Source: three-view drawing plus pictorial views. Frame: mm from the lowest corner of the part. A direction names the side the tool comes from. Round coordinates to 2 decimals unless told otherwise and drop trailing zeros. Write each loop counter-clockwise with the first axis right and the second up, starting at its lowest first coordinate (ties: lowest second). Pieces come first, ordered by that corner, then holes. Notation, with made-up numbers: (-20, -14.5) - (9, -14.5) arc R13 cw to (9, 9.5) - close; hole circle Ø7 at (8.25, 81). An arc over 180 degrees is marked (long way). Write each question's results on one line, items separated by ' | '.
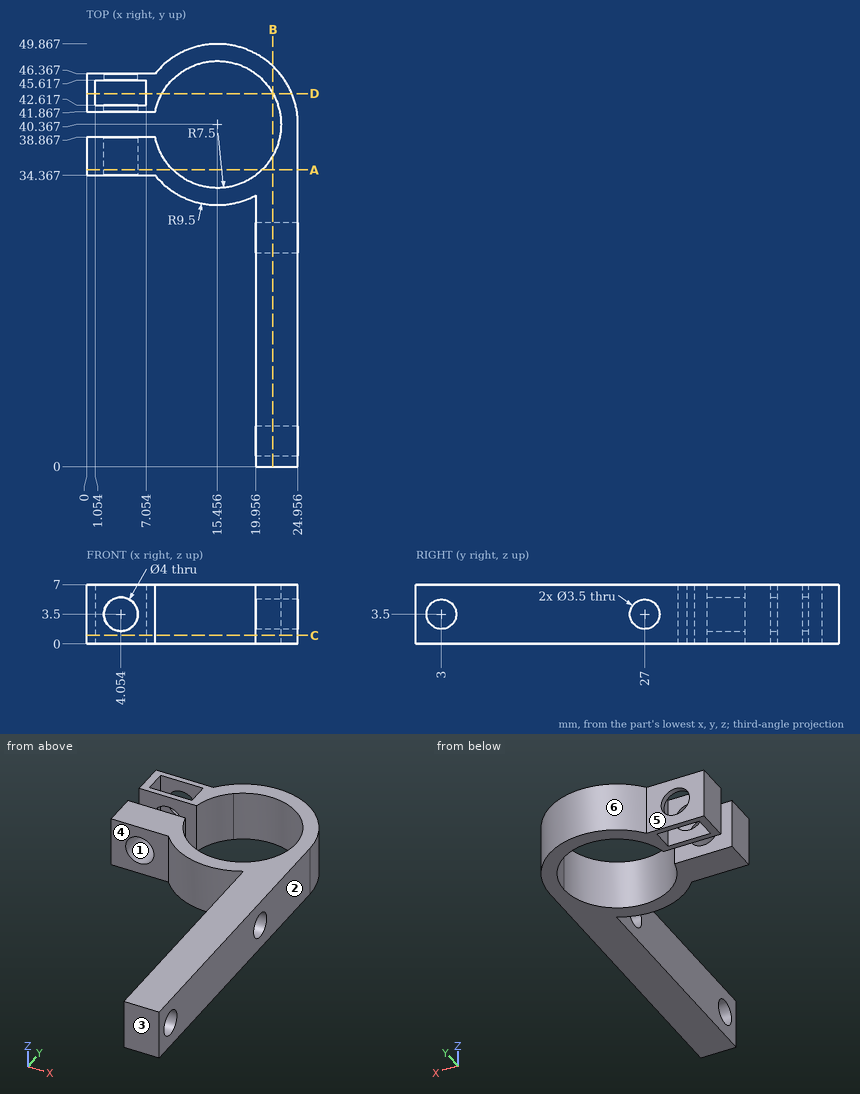
Q1. Pin query (flat end, axial travel): pin 1 (0.9 mm diameter, centred on y = 45, z = 2.5, fed in from -X); pin 2 (3.5 mm diameter, centred on x = 5, z = 3.5, fed in from -Y); pin 3 (0.9 mm diameter, centred on y = 44.5, z = 2, fed in from +X); pin 4 (4 mm diameter, centred on y = 27, z = 3.5, fed in from -X). Return the tip coordinate at first contact, or that it passes through.
Answer block:
pin 1: x = 0 | pin 2: y = 34.37 | pin 3: x = 24.21 | pin 4: x = 19.96
Q2. Section query D-D, the plane y = 44. Return loops of the section in (x, z) (1 decimal).
Answer block:
outline: (0, 0) - (1.1, 0) - (1.1, 7) - (0, 7) - close; (7.1, 0) - (8.9, 0) - (8.9, 7) - (7.1, 7) - close; (22, 0) - (24.2, 0) - (24.2, 7) - (22, 7) - close
Q3. Access query for the marked faces 4, 5 and 6. Directions: +Z, -Z, +X, -X, +Y, -Y. A direction counts if a zero-diameter tool reaches every point of the face in a straight line with its end or side. Return the directions, or none.
Answer block:
face 4: +Z, -Z, -X, -Y | face 5: +Z, -Z, -X, +Y | face 6: +Z, -Z, +Y
Q4. Mould query, pull axis X, two halves, no side actions, for the marked faces 1, 2 and 3. Classes: pulls with the +X half, pulls with the -X half, needs draft (parallel to the pull), parting line crosses it, or undercut.
Answer block:
face 1: undercut | face 2: pulls with the +X half | face 3: needs draft
Q5. Section query A-A, the plane y = 35. Return loops of the section in (x, z) (1 decimal).
Answer block:
outline: (0, 0) - (10.2, 0) - (10.2, 7) - (0, 7) - close; (20.7, 0) - (25, 0) - (25, 7) - (20.7, 7) - close; hole circle Ø4 at (4.1, 3.5)
Q6. Section query C-C, the plane z = 1. Return loops of the section in (x, y).
Answer block:
outline: (0, 34.37) - (8.09, 34.37) arc R9.5 ccw to (19.96, 32) - (19.96, 0) - (24.96, 0) - (24.96, 40.37) arc R9.5 ccw to (8.09, 46.37) - (0, 46.37) - (0, 41.87) - (8.11, 41.87) arc R7.5 cw (long way) to (8.11, 38.87) - (0, 38.87) - close; hole (1.05, 42.62) - (7.05, 42.62) - (7.05, 45.62) - (1.05, 45.62) - close
Q7. Section query B-B, the plane x = 22. Return loops of the section in (y, z), plus the area to 3 significant figures.
Answer block:
outline: (0, 0) - (36.7, 0) - (36.7, 7) - (0, 7) - close; (44.03, 0) - (47.25, 0) - (47.25, 7) - (44.03, 7) - close; hole circle Ø3.5 at (3, 3.5); hole circle Ø3.5 at (27, 3.5) | area: 260 mm2
Q8. Ray query, line 1 along X through (y, z) = (42.2, 3.5); line 2 along Y through (x, z) = (20, 4.75) (1 decimal); line 3 along Y through (x, z) = (15.25, 1.75) (1 decimal). Return the intervals inside material, ascending.
Answer block:
line 1: 0 to 2.05, 6.05 to 8.18, 22.73 to 24.78 | line 2: 0 to 1.8, 4.2 to 25.8, 28.2 to 34.4, 46.3 to 48.7 | line 3: 30.9 to 32.9, 47.9 to 49.9
